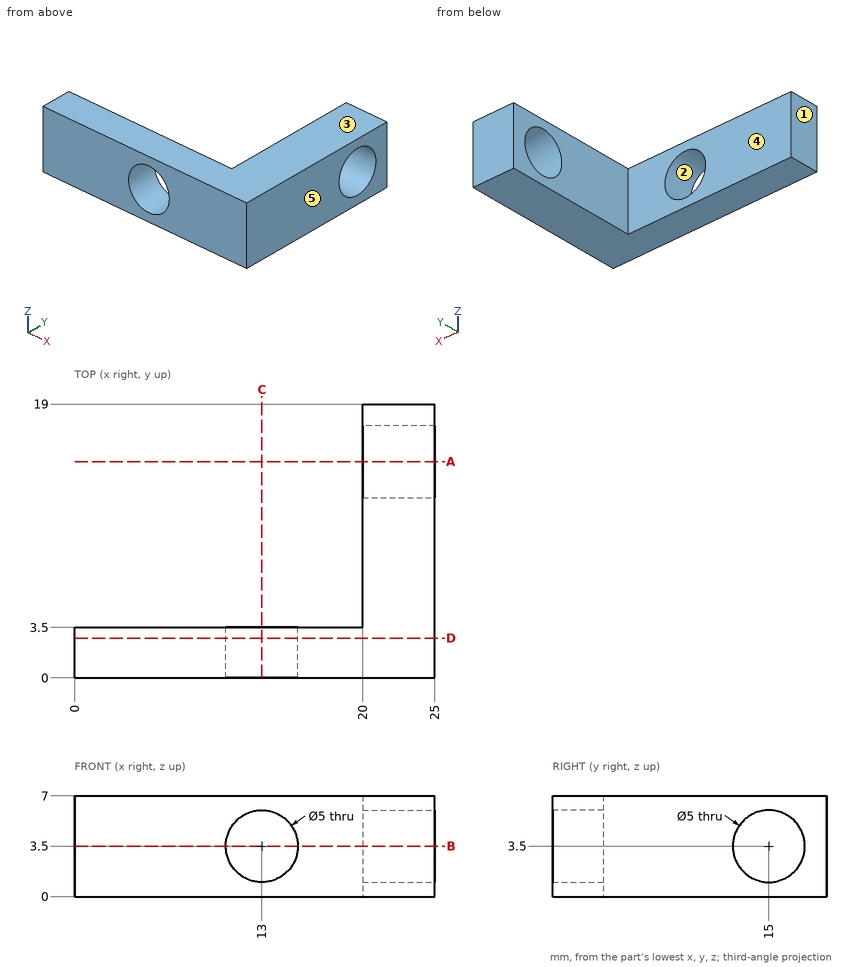
Geometry: see drawing. Coordinates: mm, zero at the bounding-box minimum. A direction names the side the tool comes from. Round coordinates to 2 decimals unless told otherwise and drop trailing zeros. Write each loop counter-clockwise with the first axis right and the second up, starting at its lowest first coordinate (ties: lowest second). Pieces come first, ordered by that corner, then holes.
Item 1: Section query B-B (z = 3.5). Return loops of the section in (x, y).
Item 2: Material intervals for L1, parallel to Z at x = 23, y = 15; L2, parallel to X at y = 1.15, z = 3.5; L3, parallel to X at y = 4.5, z = 6.25, sorted ascending.
Item 3: Set-up query: the marked faces 4 and 5. Return all of +Z, -Z, +X, -X, +Y, -Y with unobstructed straight access to the full face (end or side cutting, diameter ignored); none if empty.
Item 4: Pin query (flat end, axial travel): P1, Ø1.5, axis at x = 12.5, y = 5, coming from the +Z side. Return the tip coordinate at first contact, or that it passes through.
Item 5: Section query C-C (x = 13). Return loops of the section in (y, z).
Item 6: Section query A-A (y = 15). Return loops of the section in (x, z).
Item 7: Mould query, pull axis X, two halves, no side actions, for the marked faces 1, 2 and 3. Classes: +X half, -X half, draft (parallel to the pull), parting line (faces both ways), or undercut.
Item 8: Section query D-D (y = 2.75). Return loops of the section in (x, z), plus the area to 3 significant figures.
Completed:
1. outline: (0, 0) - (10.5, 0) - (10.5, 3.5) - (0, 3.5) - close; (15.5, 0) - (25, 0) - (25, 12.5) - (20, 12.5) - (20, 3.5) - (15.5, 3.5) - close; (20, 17.5) - (25, 17.5) - (25, 19) - (20, 19) - close
2. L1: z = 0 to 1, 6 to 7
2. L2: x = 0 to 10.5, 15.5 to 25
2. L3: x = 20 to 25
3. face 4: +Z, -Z, -X, +Y
3. face 5: +Z, -Z, +X, +Y, -Y
4. P1: passes through
5. outline: (0, 0) - (3.5, 0) - (3.5, 1) - (0, 1) - close; (0, 6) - (3.5, 6) - (3.5, 7) - (0, 7) - close
6. outline: (20, 0) - (25, 0) - (25, 1) - (20, 1) - close; (20, 6) - (25, 6) - (25, 7) - (20, 7) - close
7. face 1: -X half
7. face 2: undercut
7. face 3: draft
8. outline: (0, 0) - (25, 0) - (25, 7) - (0, 7) - close; hole circle Ø5 at (13, 3.5)
8. area: 155 mm2
